Geometry: final body of the model. Coordinates: model frame, mm. A direction names the side the tool comes from. Round coordinates to 2 decimals unless told otherwise and drop trailing zeros. Order: outer loops, then holes, each group sorted by start corner. A loop starts at its lowest first (then second) coordinate and runs counter-clockwise, first axis right, second up. Notation, with made-up numbers: M -37,45 L 19,45 A27 ccw 19,82 Z; hole C -32.75,-13.5 d7. An arc over 180 degrees is marked long. Put each result on its own line as item: value. Start each with the question number.
1) Section C-C, the plane y = 4. Count the separate pieces of the cut face and the enclosed holes in it, then the cut area to 3 significant figures.
2) Section B-B, the plane z = -1. Return loops of the section in (x, y).
3) First-contact query: P1, Ø3.5, axis at x = 7.5, z = -6, coming from the -Y side; P2, Ø7.5, axis at x = 16.5, z = -3.5, coming from the -Y side; P3, Ø1.5, axis at y = 5, z = 4.5, coming from the +X side; P4, Ø1.6, axis at x = -16, y = 7.5, coming from the -Z side. Flat tips, straight axial feed; report the tip coordinate or a pass-through.
4) Section A-A, the plane x = 0. Return loops of the section in (y, z).
5) Section D-D, the plane z = -5.5. Return loops of the section in (x, y), then the cut area to 3 significant figures.
6) Access query for faces 1 (the flat face through (2, 0, 0)), 2 (the flat face through (-13, 7, 10.3)), 3 (the cylindrical face through (-0.923, 5.774, 5.081)), 4 (the cylindrical face through (-9.361, 3.055, 9.255)), 5 (the flat face through (-13, 7, -10.3)). Directions: +Z, -Z, +X, -X, +Y, -Y. A direction counts if a zero-diameter tool reaches every point of the face in a straight line with its end or side. Return the directions, or none.
7) Draft query along X for faces 6 (the cylindrical face through (-10.3, 3, -0.1)), 7 (the flat face through (0, 8, 2)), 8 (the cylindrical face through (10.3, 3, 0.2)), 9 (the cylindrical face through (-2.11, 3.06, 10.08)). Return one class per face: pulls with the +X half, pulls with the -X half, needs draft (parallel to the pull), parting line crosses it, or undercut.
8) Material intervals for probe 1 along X at (y, z) = (5.25, 0); probe 2 along Z at (x, y) = (-6, 0.75); probe 3 along Y at (x, z) = (0, 3.25), sorted ascending. Write a range as [from, to].
from build123d import *

# Parameters (mm, degrees)
SKETCH1_R           = 1.6
BOSS_EXTRUDE1_DEPTH = 8
SKETCH3_R           = 2
CUT_EXTRUDE1_DEPTH  = 14.5
BOSS_EXTRUDE3_START = -2
BOSS_EXTRUDE3_DEPTH = 2
SKETCH5_R           = 2.25
CUT_EXTRUDE2_DEPTH  = 6.3


with BuildPart() as part:
    # Sketch1 → Boss-Extrude1 (new body)
    with BuildSketch(Plane(origin=(0, 0, 0), x_dir=(1, 0, 0), z_dir=(0, 1, 0))):
        with BuildLine():
            ThreePointArc((-9.272031939, -4.485468061), (-9.308556454, -9.308556454), (-4.485468061, -9.272031939))
            ThreePointArc((-4.485468061, -9.272031939), (0, -10.3), (4.485468061, -9.272031939))
            ThreePointArc((4.485468061, -9.272031939), (9.308556454, -9.308556454), (9.272031939, -4.485468061))
            ThreePointArc((9.272031939, -4.485468061), (10.298455819, -0.178347233), (9.421782939, 4.161731161))
            ThreePointArc((9.421782939, 4.161731161), (9.547911886, 9.547911886), (4.161731161, 9.421782939))
            ThreePointArc((4.161731161, 9.421782939), (-0.178347233, 10.298455819), (-4.485468061, 9.272031939))
            ThreePointArc((-4.485468061, 9.272031939), (-9.308556454, 9.308556454), (-9.272031939, 4.485468061))
            ThreePointArc((-9.272031939, 4.485468061), (-10.3, 0), (-9.272031939, -4.485468061))
        make_face()
        with Locations(Location((0, 0, 0), (0, 0, 270))):
            Circle(SKETCH1_R, mode=Mode.SUBTRACT)
    extrude(amount=BOSS_EXTRUDE1_DEPTH)

    # Sketch3 → Cut-Extrude1 (cut)
    with BuildSketch(Plane.XY):
        with Locations(Location((0, 4, 0), (0, 0, 180))):
            Circle(SKETCH3_R)
    extrude(amount=CUT_EXTRUDE1_DEPTH, mode=Mode.SUBTRACT)

    # Sketch4 → Boss-Extrude3 (add)
    with BuildSketch(Plane(origin=(0, 8, 0), x_dir=(1, 0, 0), z_dir=(0, 1, 0)).offset(BOSS_EXTRUDE3_START)):
        with BuildLine():
            Line((-19.439907407, 10.3), (-6.915, 10.3))
            ThreePointArc((-6.915, 10.3), (-10.052052009, 8.186664144), (-9.272031939, 4.485468061))
            ThreePointArc((-9.272031939, 4.485468061), (-10.3, 0), (-9.272031939, -4.485468061))
            ThreePointArc((-9.272031939, -4.485468061), (-10.052052009, -8.186664144), (-6.915, -10.3))
            Line((-6.915, -10.3), (-19.439907407, -10.3))
            ThreePointArc((-19.439907407, -10.3), (-22, 0), (-19.439907407, 10.3))
        make_face()
        with BuildLine():
            Line((19.256747497, 10.638499698), (6.915, 10.638499698))
            ThreePointArc((6.915, 10.638499698), (10.387480791, 8.25899671), (9.421782939, 4.161731161))
            ThreePointArc((9.421782939, 4.161731161), (10.298455819, -0.178347233), (9.272031939, -4.485468061))
            ThreePointArc((9.272031939, -4.485468061), (10.052052009, -8.186664144), (6.915, -10.3))
            Line((6.915, -10.3), (19.439907407, -10.3))
            ThreePointArc((19.439907407, -10.3), (21.999158338, 0.192438041), (19.256747497, 10.638499698))
        make_face()
    extrude(amount=BOSS_EXTRUDE3_DEPTH)

    # Sketch5 → Cut-Extrude2 (cut)
    with BuildSketch(Plane.XZ):
        with Locations(Location((-6.915, 6.915, 0), (0, 0, 270))):
            Circle(SKETCH5_R)
        with Locations(Location((6.915, 6.915, 0), (0, 0, 270))):
            Circle(SKETCH5_R)
        with Locations(Location((6.915, -6.915, 0), (0, 0, 270))):
            Circle(SKETCH5_R)
        with Locations(Location((-6.915, -6.915, 0), (0, 0, 270))):
            Circle(SKETCH5_R)
    extrude(amount=-CUT_EXTRUDE2_DEPTH, mode=Mode.SUBTRACT)


solid = part.part
Result sheet:
1. separate pieces: 1
1. enclosed holes: 4
1. area: 292 mm2
2. outline: M -21.98,6 L -10.25,6 L -10.25,0 L -1.25,0 L -1.25,8 L -21.98,8 Z; M 1.25,0 L 10.25,0 L 10.25,6 L 21.98,6 L 21.98,8 L 1.25,8 Z
3. P1: stops at y = 0
3. P2: stops at y = 6
3. P3: stops at x = 9.86
3. P4: stops at z = -10.3
4. outline: M 0,-10.3 L 8,-10.3 L 8,-1.6 L 0,-1.6 Z; M 0,1.6 L 2,1.6 L 2,10.3 L 0,10.3 Z; M 6,1.6 L 8,1.6 L 8,10.3 L 6,10.3 Z
5. outline: M -21.3,6 L -9.99,6 L -9.99,0 L -8.66,0 L -8.66,6.3 L -5.17,6.3 L -5.17,0 L 5.17,0 L 5.17,6.3 L 8.66,6.3 L 8.66,0 L 10.36,0 L 10.36,6 L 21.3,6 L 21.3,8 L -21.3,8 Z
5. area: 163 mm2
6. face 1: +Z, -Z, +X, -X, -Y
6. face 2: +Z, +X, -X, +Y, -Y
6. face 3: +Z
6. face 4: -Y
6. face 5: -Z, -X, +Y, -Y
7. face 6: pulls with the -X half
7. face 7: needs draft
7. face 8: pulls with the +X half
7. face 9: undercut
8. probe 1: x = [-10.3, -1.6], [1.6, 10.3]
8. probe 2: z = [-10.17, -8.97], [-4.86, 4.86], [8.97, 10.17]
8. probe 3: y = [0, 2], [6, 8]
